Part model, mm, in its own coordinate system. A direction names the side the tool comes from. Give positions to 0.01 mm unless a question says otherwise; leave off trailing zeros. Loops run counter-clockwise (first coordinate to the right, second up) from the corner with the lowest first, then second, coordinate; pieces in that order, holes last. Notation, with made-up numbers: (15.5, -3) -> (73.5, -3) arc R17 cw to (73.5, 3) -> close; hole circle Ø5 at (53, 21). An arc over 180 degrees is marked (long way). One line per question, with ' | ' between items.
```python
from build123d import *

# Parameters (mm, degrees)
SKETCH1_W           = 19.38
SKETCH1_H           = 26.6
BOSS_EXTRUDE1_DEPTH = 0.8
SKETCH2_W           = 0.4
SKETCH2_H           = 26.6
BOSS_EXTRUDE2_DEPTH = 2.4
SKETCH3_W           = 0.4
SKETCH3_H           = 26.6
BOSS_EXTRUDE3_DEPTH = 2.4
SKETCH4_W           = 8
SKETCH4_H           = 0.4
CUT_EXTRUDE1_DEPTH  = 27.6
SKETCH5_W           = 0.4
SKETCH5_H           = 26.6
BOSS_EXTRUDE4_DEPTH = 1.2
SKETCH6_W           = 0.4
SKETCH6_H           = 26.6
BOSS_EXTRUDE5_DEPTH = 1.2
SKETCH7_W           = 18.58
SKETCH7_H           = 0.4
BOSS_EXTRUDE6_DEPTH = 2.4
SKETCH8_W           = 2
SKETCH8_H           = 0.8
BOSS_EXTRUDE7_DEPTH = 0.8
SKETCH9_W           = 2.2470594
SKETCH9_H           = 0.8
BOSS_EXTRUDE8_DEPTH = 0.8
CUT_EXTRUDE2_DEPTH  = 11.01353


with BuildPart() as part:
    # Sketch1 → Boss-Extrude1 (new body)
    with BuildSketch(Plane.XY):
        Rectangle(SKETCH1_W, SKETCH1_H)
    extrude(amount=-BOSS_EXTRUDE1_DEPTH)

    # Sketch2 → Boss-Extrude2 (add)
    with BuildSketch(Plane(origin=(0, 0, -0.8), x_dir=(-1, 0, 0), z_dir=(0, 0, -1))):
        with Locations((-9.49, 0)):
            Rectangle(SKETCH2_W, SKETCH2_H)
    extrude(amount=BOSS_EXTRUDE2_DEPTH)

    # Sketch3 → Boss-Extrude3 (add)
    with BuildSketch(Plane(origin=(0, 0, -0.8), x_dir=(-1, 0, 0), z_dir=(0, 0, -1))):
        with Locations((9.49, 0)):
            Rectangle(SKETCH3_W, SKETCH3_H)
    extrude(amount=BOSS_EXTRUDE3_DEPTH)

    # Sketch4 → Cut-Extrude1 (cut, through all)
    with BuildSketch(Plane.XZ.offset(13.3)):
        with Locations((0, -0.2)):
            Rectangle(SKETCH4_W, SKETCH4_H)
    extrude(amount=-CUT_EXTRUDE1_DEPTH, mode=Mode.SUBTRACT)

    # Sketch5 → Boss-Extrude4 (add)
    with BuildSketch(Plane.ZY.offset(-9.29)):
        with Locations((-3, 0)):
            Rectangle(SKETCH5_W, SKETCH5_H)
    extrude(amount=BOSS_EXTRUDE4_DEPTH)

    # Sketch6 → Boss-Extrude5 (add)
    with BuildSketch(Plane(origin=(-9.29, 0, 0), x_dir=(0, 0, -1), z_dir=(1, 0, 0))):
        with Locations((3, 0)):
            Rectangle(SKETCH6_W, SKETCH6_H)
    extrude(amount=BOSS_EXTRUDE5_DEPTH)

    # Sketch7 → Boss-Extrude6 (add, through all)
    with BuildSketch(Plane(origin=(0, 0, -0.8), x_dir=(-1, 0, 0), z_dir=(0, 0, -1))):
        with Locations((0, -13.1)):
            Rectangle(SKETCH7_W, SKETCH7_H)
    extrude(amount=BOSS_EXTRUDE6_DEPTH)

    # Sketch8 → Boss-Extrude7 (add)
    with BuildSketch(Plane(origin=(0, 0, -0.8), x_dir=(-1, 0, 0), z_dir=(0, 0, -1))):
        with Locations((-4.445, 12.9)):
            Rectangle(SKETCH8_W, SKETCH8_H)
    extrude(amount=BOSS_EXTRUDE7_DEPTH)

    # Sketch9 → Boss-Extrude8 (add)
    with BuildSketch(Plane(origin=(0, 0, -0.8), x_dir=(-1, 0, 0), z_dir=(0, 0, -1))):
        with Locations((4.445, 12.9)):
            Rectangle(SKETCH9_W, SKETCH9_H)
    extrude(amount=BOSS_EXTRUDE8_DEPTH)

    # Sketch10 → Cut-Extrude2 (cut)
    with BuildSketch(Plane.ZY.offset(5.5685297)):
        Polygon((-1.6, 12.5), (-0.8, 13.3), (-1.6, 13.3), align=None)
    extrude(amount=-CUT_EXTRUDE2_DEPTH, mode=Mode.SUBTRACT)


solid = part.part
```
1) Drill centre lines: line 1 (X direction, y = -1.25, z = -0.85); line 2 (X direction, y = 4.5, z = -0.15); line 3 (Z direction, x = 8.75, y = -7.75). Where is each one in solid material? Low to high.
Found:
line 1: -9.69 to -9.29, 9.29 to 9.69 | line 2: -9.69 to -4, 4 to 9.69 | line 3: -3.2 to -2.8, -0.8 to 0
2) Pull direction Z, two halves, no side cores. Call faces 1 (the flat face through (4.4, 12.9, -1.2)), 2 (the flat face through (-9.29, 0, -2)), 3 (the flat face through (9, 0, -2.8)), 4 (the flat face through (7, 0, 0)): pulls with the +Z half, pulls with the -Z half, needs draft (parallel to the pull), parting line crosses it, or undercut.
Found:
face 1: pulls with the -Z half | face 2: undercut | face 3: undercut | face 4: pulls with the +Z half
3) Saw through at C-C (z = -2.5). Give the cut face in (x, y).
Found:
outline: (-9.69, -13.3) -> (9.69, -13.3) -> (9.69, 13.3) -> (9.29, 13.3) -> (9.29, -12.9) -> (-9.29, -12.9) -> (-9.29, 13.3) -> (-9.69, 13.3) -> close
4) Saw through at A-A (z = -1.1). Give the cut face in (x, y) (3 decimals), and give its area (3 significant figures).
Found:
outline: (-9.69, -13.3) -> (9.69, -13.3) -> (9.69, 13.3) -> (9.29, 13.3) -> (9.29, -12.9) -> (-9.29, -12.9) -> (-9.29, 13.3) -> (-9.69, 13.3) -> close; (-5.569, 12.5) -> (-3.321, 12.5) -> (-3.321, 13) -> (-5.569, 13) -> close; (3.445, 12.5) -> (5.445, 12.5) -> (5.445, 13) -> (3.445, 13) -> close | area: 30.8 mm2
5) Saw through at B-B (x = 8.75). Give the cut face in (y, z), and give its area (3 significant figures).
Found:
outline: (-13.3, -3.2) -> (13.3, -3.2) -> (13.3, -2.8) -> (-12.9, -2.8) -> (-12.9, -0.8) -> (13.3, -0.8) -> (13.3, 0) -> (-13.3, 0) -> close | area: 32.7 mm2
6) Saw through at D-D (y = -2). Give the cut face in (x, z).
Found:
outline: (-9.69, -3.2) -> (-8.09, -3.2) -> (-8.09, -2.8) -> (-9.29, -2.8) -> (-9.29, -0.8) -> (9.29, -0.8) -> (9.29, -2.8) -> (8.09, -2.8) -> (8.09, -3.2) -> (9.69, -3.2) -> (9.69, 0) -> (4, 0) -> (4, -0.4) -> (-4, -0.4) -> (-4, 0) -> (-9.69, 0) -> close
7) Pin check, flat tip, straight feed: P1, Ø6.5, axis at x = -0.5, y = -5, coming from the +Z side. Stop position of the tip, or through.
Found:
P1: z = -0.4
8) Tool access for faces 5 (the flat face through (0, 0, -0.8)), 6 (the flat face through (9.29, 0, -2)), 7 (the flat face through (-4.5, 12.9, -1.2)), 8 (the flat face through (0, 0, -0.4)): list every direction of +Z, -Z, +X, -X, +Y, -Y with a clear straight run to the whole face (end or side of a thin tool).
Found:
face 5: none | face 6: +Y | face 7: -Z, +Y | face 8: +Z, +Y, -Y
